Autodesk Inventor part; units mm, degrees
ref_plane "YZ Plane" through (0, 0, 0) normal (1, 0, 0) x (0, 1, 0)
ref_plane "XZ Plane" through (0, 0, 0) normal (0, 1, 0) x (-1, 0, 0)
ref_plane "XY Plane" through (0, 0, 0) normal (0, 0, 1) x (1, 0, 0)
sketch "Sketch1" plane through (0, 0, 0) normal (0, 1, 0) x (-1, 0, 0)
  circle A0 centre (0, 0) radius 26
  dimension "d0" = 52
extrude "Extrusion1" add sketch "Sketch1" along normal blind 200
sketch "Sketch2" plane through (0, 200, 0) normal (0, 1, 0) x (1, 0, 0)
  circle A0 centre (0, 0) radius 26
  circle A1 centre (0, 0) radius 13
  dimension "d3" = 26
extrude "Extrusion2" cut sketch "Sketch2" against normal blind 41
sketch "Sketch3" plane through (0, 0, 0) normal (0, -1, 0) x (1, 0, 0)
  circle A0 centre (0, 0) radius 13
  circle A1 centre (0, 0) radius 21.4603
  circle A2 centre (0, 0) radius 26
extrude "Extrusion3" cut sketch "Sketch3" against normal blind 39 contours A2
properties part number "spindleStandin"
Work out the finished part from the listing and answer in its coordinate system (mm). A direction names the side the tool comes from. Round coordinates to 2 decimals unless told otherwise and drop trailing zeros. Write each loop counter-clockwise with the first axis right and the second up, starting at its lowest first coordinate (ties: lowest second). Pieces come first, ordered by that corner, then holes. Notation, with made-up numbers: (36, 55.5) -> (81, 55.5) arc R7 cw to (81, 64.5) -> close; hole circle Ø8 at (10.25, 17). An arc over 180 degrees is marked (long way). Write each question's results on one line, items separated by ' | '.
Q1. Which of the six approach directions +Z, -Z, +X, -X, +Y, -Y give full straight-line access (tool end or side, diameter ignored) to faces 1 (the flat face through (0, 200, 0)), 2 (the flat face through (-6, 159, -12)), 3 (the cylindrical face through (-15.82, 19.23, 14.5))?
Data:
face 1: +Z, -Z, +X, -X, +Y | face 2: +Y | face 3: -Y
Q2. Section D-D, the plane z = -16 is taken. Write down the section's boundary in (x, y), then the cut area to 3 significant figures.
Data:
outline: (-20.49, 39) -> (-14.3, 39) -> (-14.3, 0) -> (14.3, 0) -> (14.3, 39) -> (20.49, 39) -> (20.49, 159) -> (-20.49, 159) -> close | area: 6,030 mm^2
Q3. Flat-ended cylindrical pins translate along their axes: P1, Ø1, axis at x = -15, z = 1.5, coming from the +Y side; P2, Ø4, axis at y = 76.5, z = 10.5, coming from the -X side; P3, Ø3, axis at x = -15, y = 176, coming from the -Z side; P4, Ø3, axis at y = 110, z = -2.5, coming from the +X side. Find the tip coordinate at first contact, or state that the pin passes through.
Data:
P1: y = 159 | P2: x = -24.57 | P3: through | P4: x = 25.98
Q4. Section B-B, the plane z = 0 is taken. Write down the section's boundary in (x, y), then the cut area to 3 significant figures.
Data:
outline: (-26, 39) -> (-21.46, 39) -> (-21.46, 0) -> (21.46, 0) -> (21.46, 39) -> (26, 39) -> (26, 159) -> (13, 159) -> (13, 200) -> (-13, 200) -> (-13, 159) -> (-26, 159) -> close | area: 8,980 mm^2
Q5. Straight lines are drawn through the part: line 1 along Y through (x, z) = (-12.5, 11); line 2 along Y through (x, z) = (20, -8); line 3 along X through (y, z) = (48, -6). For each, find the intervals that lie inside material, in ascending order. Write a range as [from, to].
Data:
line 1: [0, 159] | line 2: [39, 159] | line 3: [-25.3, 25.3]
Q6. Section A-A, the plane x = 0 is taken. Write down the section's boundary in (y, z), then the cut area to 3 significant figures.
Data:
outline: (0, -21.46) -> (39, -21.46) -> (39, -26) -> (159, -26) -> (159, -13) -> (200, -13) -> (200, 13) -> (159, 13) -> (159, 26) -> (39, 26) -> (39, 21.46) -> (0, 21.46) -> close | area: 8,980 mm^2
Q7. Section C-C, the plane y = 110.5 is taken. Write down the section's boundary in (x, z), then the cut area to 3 significant figures.
Data:
outline: circle Ø52 at (0, 0) | area: 2,120 mm^2
